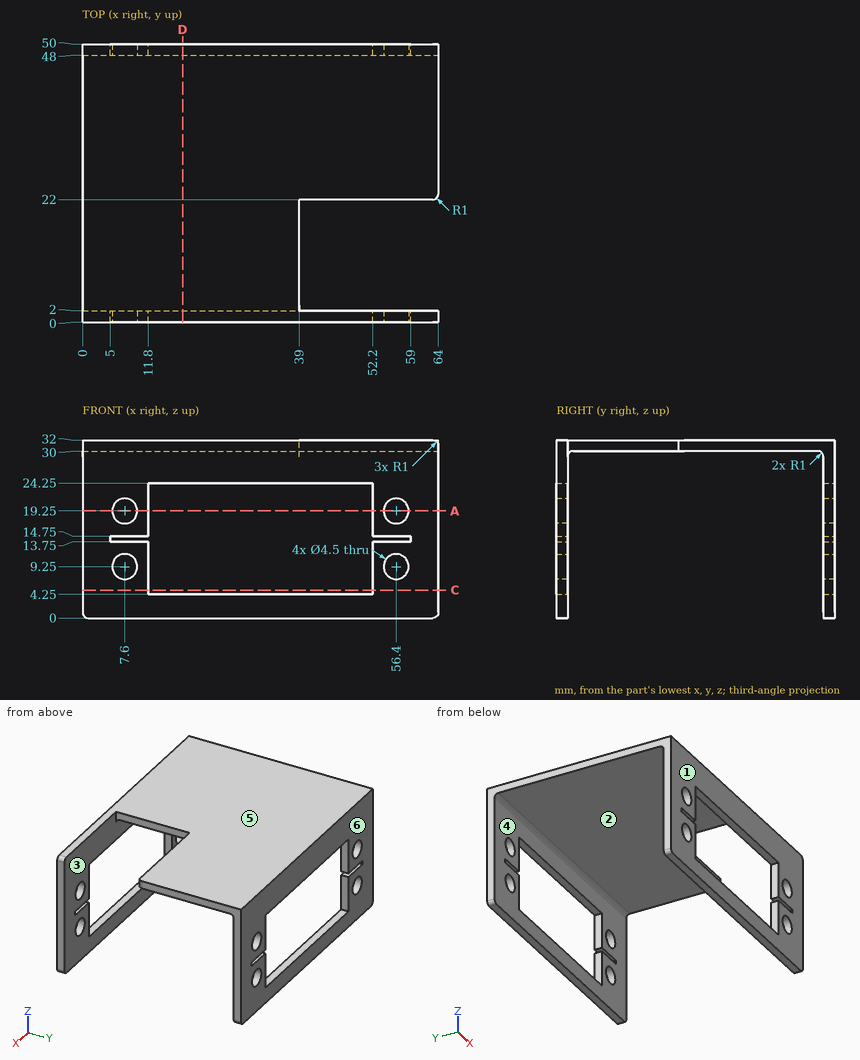
Source: three-view drawing plus pictorial views. Frame: mm from the lowest corner of the part. A direction names the side the tool comes from. Give positions to 0.01 mm unless a question says otherwise; leave off trailing zeros. Loops run counter-clockwise (first coordinate to the right, second up) from the corner with the lowest first, then second, coordinate; pieces in that order, holes last. Notation, with made-up numbers: M -8,-28.5 L 14,-28.5 A21 cw 14,-13.5 Z; hole C -19,29.5 d10. An arc over 180 degrees is marked long. Put each result on its own line as item: value.
Q1. Pin query (flat end, axial travel): P1, Ø5, axis at x = 13.5, y = 5.5, coming from the -Z side; P2, Ø0.9, axis at y = 16, z = 31, coming from the +X side. Return the tip coordinate at first contact, or that it passes through.
Response values:
P1: stops at z = 30
P2: stops at x = 39
Q2. Section C-C (z = 5). Return the cut outline in (x, y), and give its area (3 significant figures).
Response values:
outline: M 0,0 L 11.8,0 L 11.8,2 L 0,2 Z; M 0,48 L 11.8,48 L 11.8,50 L 0,50 Z; M 52.2,0 L 64,0 L 64,2 L 52.2,2 Z; M 52.2,48 L 64,48 L 64,50 L 52.2,50 Z
area: 94.4 mm²
Q3. Line query: probe 1 along X at (y, z) = (0.55, 19.25); probe 2 along Z at (x, y) = (7.6, 0.9); probe 3 along Y at (x, z) = (31, 26). Output: solid intervals per line, ascending. Write a range as [from, to].
Response values:
probe 1: x = [0, 5.35], [9.85, 11.8], [52.2, 54.15], [58.65, 64]
probe 2: z = [0, 7], [11.5, 13.75], [14.75, 17], [21.5, 32]
probe 3: y = [0, 2], [48, 50]
Q4. Reachability of the marked faces 1 and 2 from +Z, -Z, +X, -X, +Y, -Y: full face, straight path, thin tool, end or side. Return the list, or none.
Response values:
face 1: +Z, -Z, +X, -X, -Y
face 2: -Z, +X, -X
Q5. Mould query, pull axis Y, two halves, no side actions, for the marked faces 3, 4, 5 and 6. Classes: released by +Y, released by -Y, zero draft, split by the parting line, or undercut.
Response values:
face 3: undercut
face 4: undercut
face 5: zero draft
face 6: released by +Y
Q6. Section A-A (z = 19.25). Count the separate pieces of the cut face and the enclosed holes in it, and give its area (3 significant figures).
Response values:
separate pieces: 8
enclosed holes: 0
area: 58.4 mm²
Q7. Section D-D (x = 18). Return the cut outline in (y, z), and give its area (3 significant figures).
Response values:
outline: M 0,0 L 2,0 L 2,4.25 L 0,4.25 Z; M 0,24.25 L 2,24.25 L 2,29 A1 cw 3,30 L 47,30 A1 cw 48,29 L 48,24.25 L 50,24.25 L 50,32 L 0,32 Z; M 48,0 L 50,0 L 50,4.25 L 48,4.25 Z
area: 140 mm²
